from build123d import *

# Parameters (mm, degrees)
SKETCH1_R           = 5
BOSS_EXTRUDE1_DEPTH = 4


with BuildPart() as part:
    # Sketch1 → Boss-Extrude1 (new body)
    with BuildSketch(Plane.XY):
        with BuildLine():
            Line((75, -7.5), (-75, -7.5))
            ThreePointArc((-75, -7.5), (-82.5, 0), (-75, 7.5))
            Line((-75, 7.5), (75, 7.5))
            ThreePointArc((75, 7.5), (82.5, 0), (75, -7.5))
        make_face()
        with Locations((75, 0)):
            Circle(SKETCH1_R, mode=Mode.SUBTRACT)
        with Locations(Location((-75, 0, 0), (0, 0, 180))):
            Circle(SKETCH1_R, mode=Mode.SUBTRACT)
        with BuildLine():
            Line((-0.965077795, 3.3973761), (-14.211482552, 1.988787352))
            ThreePointArc((-14.211482552, 1.988787352), (-16, 0), (-14.211482552, -1.988787352))
            Line((-14.211482552, -1.988787352), (-0.965077795, -3.3973761))
            ThreePointArc((-0.965077795, -3.3973761), (0.000431807, -3.453017023), (0.966800983, -3.415131426))
            Line((0.966800983, -3.415131426), (17.174893203, -1.992338417))
            ThreePointArc((17.174893203, -1.992338417), (19, 0), (17.174893203, 1.992338417))
            Line((17.174893203, 1.992338417), (0.966800983, 3.415131426))
            ThreePointArc((0.966800983, 3.415131426), (0.000431807, 3.453017023), (-0.965077795, 3.3973761))
        make_face(mode=Mode.SUBTRACT)
    extrude(amount=BOSS_EXTRUDE1_DEPTH)


solid = part.part
Verification items for the finished model (mm, model axes). A direction names the side the tool comes from. Coordinates: 2 decimals unless noted, no trailing zeros. Order: outer loops, then holes, each group sorted by start corner. A loop starts at its lowest first (then second) coordinate and runs counter-clockwise, first axis right, second up. Notation, with made-up numbers: M -13.75,54.5 L 10.25,54.5 A18 cw 10.25,85.5 Z; hole C -21.75,42.5 d8. An arc over 180 degrees is marked long. One line per item, written item: value. Start each with the question number.
Item 1: Sectioned sample at B-B on z = 1.85. Record the cut outline in (x, y), then the cut area to 3 significant figures.
Item 2: Depth check by flat-ended pin: P1, Ø1.5, axis at y = 1, z = 3, coming from the -X side. Enter the tip coordinate at first touch or a pass-through.
Item 3: Access from +Z, -Z, +X, -X, +Y, -Y to the whole of each face (thin tool, end or side, straight path). Record for faces 4 (the flat face through (-1, 7.5, 2)), 5 (the flat face through (-7.681, -2.683, 1.972)).
Item 4: Mould release check, pull along X, two halves, no side actions. Record for faces 1 (the cylindrical face through (82.5, 0.16, 1.97)), 2 (the cylindrical face through (-79.619, 1.915, 1.972)), 3 (the flat face through (1, 5, 4)): pulls with the +X half, pulls with the -X half, needs draft (parallel to the pull), parting line crosses it, or undercut.
Item 5: Sectioned sample at A-A on y = 0. Record the cut outline in (x, z), then the cut area to 3 significant figures.
Item 6: Thickness scan on probe 1 along X at (y, z) = (-0.25, 2.6); probe 2 along X at (y, z) = (1.25, 0.8); probe 3 along Y at (x, z) = (-75, 0.9). Record the ranges inside material, lowest first.
Calculated:
1. outline: M -75,-7.5 L 75,-7.5 A7.5 ccw 75,7.5 L -75,7.5 A7.5 ccw Z; hole C -75,0 d10; hole M -14.21,-1.99 L -0.97,-3.4 A10 ccw 0.97,-3.42 L 17.17,-1.99 A2 ccw 17.17,1.99 L 0.97,3.42 A10 ccw -0.97,3.4 L -14.21,1.99 A2 ccw Z; hole C 75,0 d10
1. area: 2,090 mm^2
2. P1: x = -82.5
3. face 4: +Z, -Z, +X, -X, +Y
3. face 5: +Z, -Z
4. face 1: pulls with the +X half
4. face 2: undercut
4. face 3: needs draft
5. outline: M -82.5,0 L -80,0 L -80,4 L -82.5,4 Z; M -70,0 L -16,0 L -16,4 L -70,4 Z; M 19,0 L 70,0 L 70,4 L 19,4 Z; M 80,0 L 82.5,0 L 82.5,4 L 80,4 Z
5. area: 440 mm^2
6. probe 1: -82.5 to -79.99, -70.01 to -15.98, 18.98 to 70.01, 79.99 to 82.5
6. probe 2: -82.4 to -79.84, -70.16 to -15.56, 18.56 to 70.16, 79.84 to 82.4
6. probe 3: -7.5 to -5, 5 to 7.5
